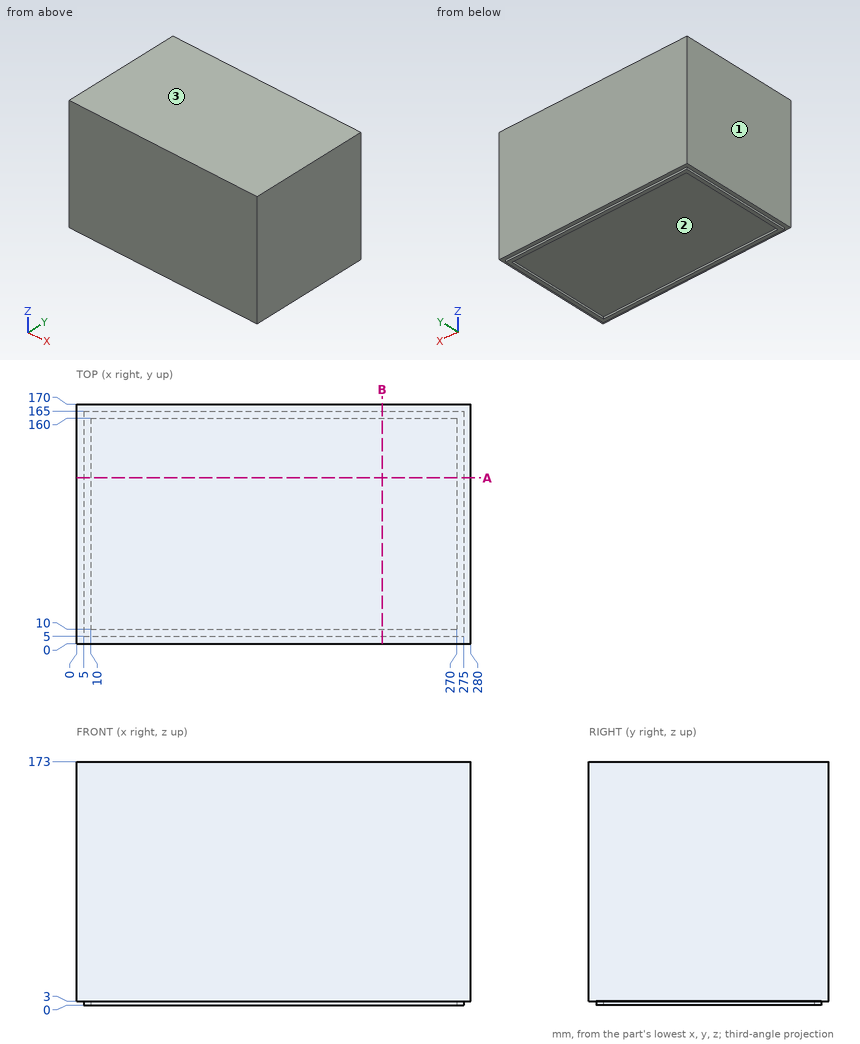
Study the drawing (mm; zero at the part's minimum x, y, z) and answer. Coordinates: 2 decimals unless noted, no trailing zeros. Order: outer loops, then holes, each group sorted by start corner. A loop starts at its lowest first (then second) coordinate and runs counter-clockwise, first axis right, second up. Notation, with made-up numbers: M 57,43.25 L 73,43.25 A26 ccw 73,59.25 Z; hole C -5,65 d5. An arc over 180 degrees is marked long. Use CSV: the item, a comma, the result in double quotes.
Q1. Determine the mould class of the marked faces 1, 2 and 3 for opening direction X: pulls with the +X half, pulls with the -X half, needs draft (parallel to the pull), parting line crosses it, or undercut.
Here are the results:
face 1,"pulls with the -X half"
face 2,"undercut"
face 3,"needs draft"
Q2. Section A-A (y = 117.5) is taken. Determine the outline of the cut face in (x, z), then the cut area to 3 significant figures.
Here are the results:
outline,"M 0,3 L 5,3 L 5,0 L 10,0 L 10,3 L 270,3 L 270,0 L 275,0 L 275,3 L 280,3 L 280,173 L 0,173 Z"
area,"47,600 mm2"
Q3. A straight line is drawn through the part: L1, parallel to Z at x = 229, y = 100.5. Find the intervals that lie inside material, in ascending order.
Here are the results:
L1,"3 to 173"
Q4. Given pin 1 Ø1.5 at (x, z) = (114, 1.5) entering from +Y; pin 2 Ø5 at (x, z) = (65, 117) entering from -Y; pin 3 Ø0.9 at (y, z) = (98, 1) entering from +X; pin 4 Ø3 at (x, y) = (93.5, 58) entering from -Z, each flat-ended and moving along its own axis, determine where each tip first touches the part or whether it passes through.
Here are the results:
pin 1,"y = 165"
pin 2,"y = 0"
pin 3,"x = 275"
pin 4,"z = 3"
Q5. Section B-B (x = 217) is taken. Determine the outline of the cut face in (y, z), then the cut area to 3 significant figures.
Here are the results:
outline,"M 0,3 L 5,3 L 5,0 L 10,0 L 10,3 L 160,3 L 160,0 L 165,0 L 165,3 L 170,3 L 170,173 L 0,173 Z"
area,"28,900 mm2"
